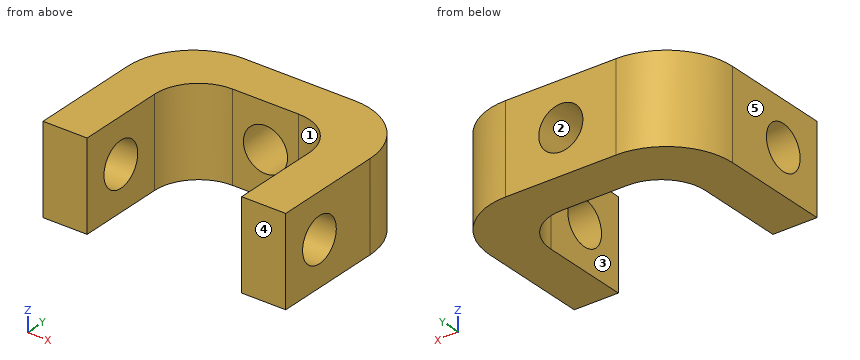
Autodesk Inventor part; units mm, degrees
ref_plane "YZ Plane" through (0, 0, 0) normal (1, 0, 0) x (0, 1, 0)
ref_plane "XZ Plane" through (0, 0, 0) normal (0, 1, 0) x (-1, 0, 0)
ref_plane "XY Plane" through (0, 0, 0) normal (0, 0, 1) x (1, 0, 0)
sketch "Sketch1" plane through (0, 0, 0) normal (0, 0, 1) x (1, 0, 0)
  line L0 (0, 0) -> (10, 0)
  line L1 (10, 0) -> (10, 30)
  line L2 (10, 30) -> (45, 30)
  line L3 (45, 30) -> (45, 0)
  line L4 (45, 0) -> (55, 0)
  line L5 (55, 0) -> (55, 40)
  line L6 (55, 40) -> (0, 40)
  line L7 (0, 40) -> (0, 0)
  dimension "d0" = 10
  dimension "d1" = 35
  dimension "d2" = 10
  dimension "d3" = 40
  dimension "d4" = 10
extrude "Extrusion1" add sketch "Sketch1" along normal blind 20
sketch "Sketch2" plane through (55, 0, 0) normal (1, 0, 0) x (0, 0, -1)
  circle A0 centre (-10, 10) radius 5
  line L0 (0, 0) -> (0, 40)
  line L1 (0, 0) -> (0, 40)
  line L2 (0, 40) -> (-20, 40)
  line L3 (-20, 0) -> (-20, 40)
  line L4 (0, 0) -> (-20, 0)
  dimension "d7" = 10
  dimension "d8" = 10
  dimension "d9" = 20
  dimension "d10" = 10
extrude "Extrusion2" cut sketch "Sketch2" against normal through all contours A0
sketch "Sketch3" plane through (0, 40, 0) normal (0, 1, 0) x (1, 0, 0)
  line L0 (55, 0) -> (0, 0)
  line L1 (0, 0) -> (0, -20)
  line L2 (55, -20) -> (0, -20)
  line L3 (55, 0) -> (55, -20)
  circle A0 centre (27.5, -10) radius 5
  point P0 (0, 0)
  dimension "d13" = 55
  dimension "d14" = 10
  dimension "d15" = 27.5
  dimension "d16" = 20
  dimension "d17" = 10
extrude "Extrusion3" cut sketch "Sketch3" against normal up to next contours A0
fillet "Fillet2" radius 10 2 edges at (10, 30, 10) (45, 30, 10)
fillet "Fillet4" radius 15 2 edges at (0, 40, 10) (55, 40, 10)
equation "\"d8\" = 0.5 * d9"
equation "\"d15\" = 0.5 * d13"
equation "\"d17\" = 0.5 * d16"
properties part number "EE_base_connection" material "Acetal Resin, Black"
Build history of the part. All positions in model axes, mm. Face numbers are marked on the shaded views. A direction names the side the tool comes from. Give positions to 0.01 mm unless a question says otherwise; leave off trailing zeros. Loops run counter-clockwise (first coordinate to the right, second up) from the corner with the lowest first, then second, coordinate; pieces in that order, holes last. Notation, with made-up numbers: (-39.5, 7.25) -> (-2.5, 7.25) arc R8 ccw to (-2.5, 14.25) -> close; hole circle Ø5 at (-13.5, 10.25). An arc over 180 degrees is marked (long way). One line per question, with ' | ' between items. Start each with the question number.
1) Cut at A-A (x = 27.5). Give the cut face in (y, z).
2) Cut at C-C (y = 10). Give the cut face in (x, z), plus the area to 3 significant figures.
3) Cut at D-D (z = 17.75). Give the cut face in (x, y).
4) 3-axis set-ups, long thin cutter, end or side, ignore diameter. For the marked faces 1 and 2: which of +Z, -Z, +X, -X, +Y, -Y reach the whole face in a straight line?
5) Pin check, flat tips, straight feed: pin 1 (3 mm diameter, centred on y = 8, z = 8.5, fed in from +X); pin 2 (7.5 mm diameter, centred on x = 26, z = 5, fed in from -Y); pin 3 (10 mm diameter, centred on x = 16.5, z = 9.5, fed in from -Y). Stop position of each tip, or through.
6) Probe L1, parallel to X at y = 16.5, z = 8.25; L2, parallel to Y at x = 35, z = 9; L3, parallel to Y at x = 4, z = 10. List the from-to ranges inside material, lowest first.
7) Cut at B-B (z = 10). Give the cut face in (x, y), plus the area to 3 significant figures.
8) Two-plate mould, pull along X, no slides. Class the marked faces 3, 4 and 5: released by +X, released by -X, zero draft, split by the parting line, or undercut.
Return value:
1) outline: (30, 0) -> (40, 0) -> (40, 5) -> (30, 5) -> close; (30, 15) -> (40, 15) -> (40, 20) -> (30, 20) -> close
2) outline: (0, 0) -> (10, 0) -> (10, 5) -> (0, 5) -> close; (0, 15) -> (10, 15) -> (10, 20) -> (0, 20) -> close; (45, 0) -> (55, 0) -> (55, 5) -> (45, 5) -> close; (45, 15) -> (55, 15) -> (55, 20) -> (45, 20) -> close | area: 200 mm^2
3) outline: (0, 0) -> (10, 0) -> (10, 20) arc R10 cw to (20, 30) -> (35, 30) arc R10 cw to (45, 20) -> (45, 0) -> (55, 0) -> (55, 25) arc R15 ccw to (40, 40) -> (15, 40) arc R15 ccw to (0, 25) -> close
4) face 1: +Z, -Z, -Y | face 2: +Y, -Y
5) pin 1: through | pin 2: y = 30 | pin 3: y = 25.27
6) L1: 0 to 10, 45 to 55 | L2: 30 to 40 | L3: 0 to 5, 15 to 35.2
7) outline: (0, 0) -> (10, 0) -> (10, 5) -> (0, 5) -> close; (0, 15) -> (10, 15) -> (10, 20) arc R10 cw to (20, 30) -> (22.5, 30) -> (22.5, 40) -> (15, 40) arc R15 ccw to (0, 25) -> close; (32.5, 30) -> (35, 30) arc R10 cw to (45, 20) -> (45, 15) -> (55, 15) -> (55, 25) arc R15 ccw to (40, 40) -> (32.5, 40) -> close; (45, 0) -> (55, 0) -> (55, 5) -> (45, 5) -> close | area: 796 mm^2
8) face 3: undercut | face 4: zero draft | face 5: released by -X
